Part model, mm, in its own coordinate system. Give positions to 0.01 mm unless a question says otherwise; leave off trailing zeros. Order: outer loops, then holes, each group sorted by start corner. A loop starts at its lowest first (then second) coordinate and runs counter-clockwise, first axis right, second up. Notation, with made-up numbers: M -9.5,-22.5 L 45.5,-22.5 A10 ccw 45.5,-16.5 Z; hole C 23.5,-8 d8. An arc over 180 degrees is marked long. Return JSON: item names as keys, results as strings.
from build123d import *

# Parameters (mm, degrees)
F0_W     = 327.025
F0_H     = 381
F1_DEPTH = 19.05
F2_W     = 4.7625
F2_H     = 9.525
F3_DEPTH = 327.025
F4_W     = 38.1
F4_H     = 9.525
F4_W_2   = 44.45
F5_DEPTH = 9.525
F6_W     = 276.225
F6_H     = 25.4
F7_DEPTH = 9.525


with BuildPart() as f1:
    # F0 (on Right) → F1 (new body)
    with BuildSketch(Plane.YZ):
        with Locations((163.5125, 190.5)):
            Rectangle(F0_W, F0_H)
    extrude(amount=F1_DEPTH)

    # F2 (on Front) → F3 (cut, through all)
    with BuildSketch(Plane.XZ):
        with Locations((2.38125, 376.2375)):
            Rectangle(F2_W, F2_H)
        with Locations((16.66875, 376.2375)):
            Rectangle(F2_W, F2_H)
        with Locations((2.38125, 4.7625)):
            Rectangle(F2_W, F2_H)
        with Locations((16.66875, 4.7625)):
            Rectangle(F2_W, F2_H)
    extrude(amount=-F3_DEPTH, mode=Mode.SUBTRACT)

    # F4 (on face) → F5 (cut, through all)
    with BuildSketch(Plane.YZ.offset(14.2875)):
        with Locations((19.05, 376.2375)):
            Rectangle(F4_W, F4_H)
        with Locations((19.05, 4.7625)):
            Rectangle(F4_W, F4_H)
        with Locations((304.8, 376.2375)):
            Rectangle(F4_W_2, F4_H)
        with Locations((304.8, 4.7625)):
            Rectangle(F4_W_2, F4_H)
    extrude(amount=-F5_DEPTH, mode=Mode.SUBTRACT)

    # F6 (on face) → F7 (cut)
    with BuildSketch(Plane(origin=(0, 0, 0), x_dir=(0, -1, 0), z_dir=(-1, 0, 0))):
        with Locations((-163.5125, 301.625)):
            Rectangle(F6_W, F6_H)
        with Locations((-163.5125, 149.225)):
            Rectangle(F6_W, F6_H)
    extrude(amount=-F7_DEPTH, mode=Mode.SUBTRACT)


solid = f1.part
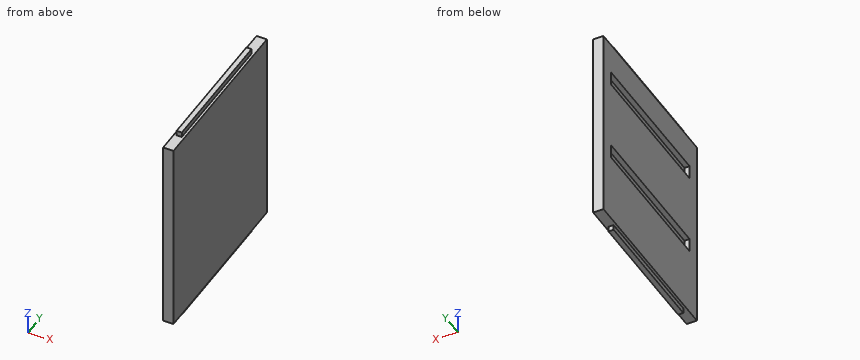
Q1. Band-saw the part on B-B (y = 295). Give the cut face in (x, z) (3 decimals), then the cut area to 3 significant figures.
Established:
{"outline": "M 0,9.525 L 19.05,9.525 L 19.05,371.475 L 0,371.475 L 0,314.325 L 9.525,314.325 L 9.525,288.925 L 0,288.925 L 0,161.925 L 9.525,161.925 L 9.525,136.525 L 0,136.525 Z", "area": "6,410 mm²"}
Q2. Pin check, flat tips, straight feed: pin 1 (7.5 mm diameter, centred on y = 221.5, z = 144, fed in from -X) (3 decimals); pin 2 (2 mm diameter, centred on x = 8.5, y = 289.5, fed in from +Z) (3 decimals); pin 3 (5 mm diameter, centred on y = 167, z = 377, fed in from -X). Stop position of each tip, or through.
Established:
{"pin 1": "stops at x = 9.525", "pin 2": "stops at z = 371.475", "pin 3": "stops at x = 4.76"}
Q3. Band-saw the part on A-A (z = 147). Give the cut face in (x, y) (3 decimals), then the cut area to 3 significant figures.
Established:
{"outline": "M 0,0 L 19.05,0 L 19.05,327.025 L 0,327.025 L 0,301.625 L 9.525,301.625 L 9.525,25.4 L 0,25.4 Z", "area": "3,600 mm²"}
Q4. Probe line 1 along Z through (x, y) = (2, 246.5) (3 decimals); line 2 along Z through (x, y) = (7.5, 98) (3 decimals); line 3 along Z through (x, y) = (15, 170) (3 decimals). List the from-to ranges inside material, lowest first.
Established:
{"line 1": "z = 9.525 to 136.525, 161.925 to 288.925, 314.325 to 371.475", "line 2": "z = 0 to 136.525, 161.925 to 288.925, 314.325 to 381", "line 3": "z = 9.525 to 371.475"}
